```python
from build123d import *

# Parameters (mm, degrees)
SKETCH1_R           = 10.789707568
BOSS_EXTRUDE1_DEPTH = 25.4
BOSS_EXTRUDE2_DEPTH = 3.056759297
SKETCH3_W           = 31.75
SKETCH3_H           = 65.18759886
BOSS_EXTRUDE3_DEPTH = 15.463355349
SKETCH4_W           = 31.75
SKETCH4_H           = 0.86411943
BOSS_EXTRUDE4_DEPTH = 44.925321362
SKETCH5_W           = 31.75
SKETCH5_H           = 6.825321362
BOSS_EXTRUDE5_DEPTH = 25.4


with BuildPart() as part:
    # Sketch1 → Boss-Extrude1 (new body)
    with BuildSketch(Plane.YZ):
        with Locations(Location((0, 0, 0), (0, 0, 270))):
            Circle(SKETCH1_R)
    extrude(amount=BOSS_EXTRUDE1_DEPTH)

    # Sketch2 → Boss-Extrude2 (add)
    with BuildSketch(Plane(origin=(0, 0, 0), x_dir=(0, -1, 0), z_dir=(-1, 0, 0))):
        with BuildLine():
            Line((2.54, -10.789707568), (-2.54, -10.789707568))
            ThreePointArc((-2.54, -10.789707568), (-9.724204897, -7.813912465), (-12.7, -0.629707568))
            Line((-12.7, -0.629707568), (-12.7, 14.610292432))
            Line((-12.7, 14.610292432), (12.7, 14.610292432))
            Line((12.7, 14.610292432), (12.7, -0.629707568))
            ThreePointArc((12.7, -0.629707568), (9.724204897, -7.813912465), (2.54, -10.789707568))
        make_face()
    extrude(amount=BOSS_EXTRUDE2_DEPTH)

    # Sketch3 → Boss-Extrude3 (add)
    with BuildSketch(Plane.XY.offset(14.610292432)):
        with Locations((12.818240703, 0)):
            Rectangle(SKETCH3_W, SKETCH3_H)
    extrude(amount=BOSS_EXTRUDE3_DEPTH)


with BuildPart() as body_2:
    # Sketch4 → Boss-Extrude4 (new body)
    with BuildSketch(Plane.XY.offset(30.073647781)):
        with Locations((12.818240703, 32.161739715)):
            Rectangle(SKETCH4_W, SKETCH4_H)
    extrude(amount=BOSS_EXTRUDE4_DEPTH)

    # Sketch5 → Boss-Extrude5 (add)
    with BuildSketch(Plane.XZ.offset(-31.72968)):
        with Locations((12.818240703, 71.586308462)):
            Rectangle(SKETCH5_W, SKETCH5_H)
    extrude(amount=BOSS_EXTRUDE5_DEPTH)


with BuildPart() as body_3:
    # Mirror1: mirrored copy
    add(body_2.part.mirror(Plane.ZX))


with BuildPart() as body_2_1:
    add(body_2.part)

    # Combine1: union part, body 3
    add(part.part)
    add(body_3.part)


solid = body_2_1.part
```
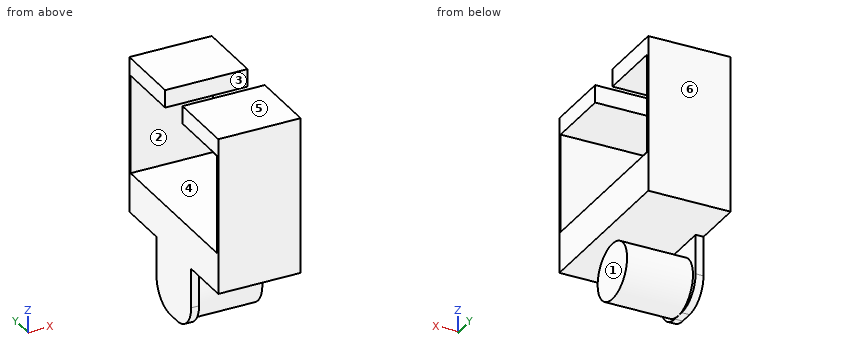
Can you work these out from the model? Positions are in its coordinate system, mm. Face numbers are marked on the shaded views. A direction names the side the tool comes from. Round coordinates to 2 decimals unless told otherwise and drop trailing zeros. Loops run counter-clockwise (first coordinate to the right, second up) from the corner with the lowest first, then second, coordinate; pieces in that order, holes last. Notation, with made-up numbers: (16, 23.5) -> (29, 23.5) arc R12 cw to (29, 37.5) -> close; hole circle Ø7 at (87.25, 59). An arc over 180 degrees is marked (long way). One line per item, written item: value. Start each with the question number.
1. If we section it at B-B, the plane x = 12.5: Write out the boundary of the cut face in (y, z), then the cut area to 3 significant figures.
2. For the marked faces 1, 2 and 3, which set-ups out of +Z, -Z, +X, -X, +Y, -Y let a thin tool reach every point of the face, with its end or its side?
3. If we mould it in two halves opening along Y, with no side actions, what happens to the marked faces 4, 5 and 6? For each: pulls with the +Y half, pulls with the -Y half, needs draft (parallel to the pull), parting line crosses it, or undercut.
4. If I drill on probe 1 along Y at (x, z) = (23.5, 64.5); probe 2 along Z at (x, y) = (1, 12.5); probe 3 along Z at (x, y) = (13, 7), over which ranges is the centre line in solid material (lowest first)?
5. If we section it at A-A, the plane y = -25: Write out the boundary of the cut face in (x, z).
6. For pin 1 (5 mm diameter, centred on x = 12.5, y = 14, fed in from -Z); pin 2 (9.5 mm diameter, centred on x = 11.5, y = 5, fed in from +Z); pin 3 (2 mm diameter, centred on x = 1.5, y = -0.5, fed in from +Z); pin 4 (5 mm diameter, centred on y = -17, z = 0, fed in from -X) (3 decimals), each with a flat end and sliding along its axis, tell me the tip position at first contact or that it passes through.
7. If we section it at C-C, the plane z = 46.5: Write out the boundary of the cut face in (x, y), then the cut area to 3 significant figures.
Calculated:
1. outline: (-32.59, 14.61) -> (32.59, 14.61) -> (32.59, 75) -> (6.33, 75) -> (6.33, 68.17) -> (31.73, 68.17) -> (31.73, 30.07) -> (-31.73, 30.07) -> (-31.73, 68.17) -> (-6.33, 68.17) -> (-6.33, 75) -> (-32.59, 75) -> close; circle Ø21.58 at (0, 0)
1. area: 1,800 mm²
2. face 1: -Z, +X, +Y, -Y
2. face 2: +X, -X
2. face 3: +Z, +X, -X
3. face 4: undercut
3. face 5: needs draft
3. face 6: pulls with the +Y half
4. probe 1: y = -32.59 to -31.73, 31.73 to 32.59
4. probe 2: z = 14.61 to 30.07, 68.17 to 75
4. probe 3: z = -8.21 to 8.21, 14.61 to 30.07, 68.17 to 75
5. outline: (-3.06, 14.61) -> (28.69, 14.61) -> (28.69, 30.07) -> (-3.06, 30.07) -> close; (-3.06, 68.17) -> (28.69, 68.17) -> (28.69, 75) -> (-3.06, 75) -> close
6. pin 1: stops at z = 14.61
6. pin 2: stops at z = 75
6. pin 3: stops at z = 30.07
6. pin 4: passes through
7. outline: (-3.06, -32.59) -> (28.69, -32.59) -> (28.69, -31.73) -> (-3.06, -31.73) -> close; (-3.06, 31.73) -> (28.69, 31.73) -> (28.69, 32.59) -> (-3.06, 32.59) -> close
7. area: 54.9 mm²
